For this review, take the finished solid that the model builds, in its own axes (mm). Give positions to 0.01 mm unless a question says otherwise; leave off trailing zeros. Order: outer loops, then holes, each group sorted by start corner. A loop starts at its lowest first (then second) coordinate and runs counter-clockwise, first axis right, second up. Notation, with made-up numbers: (49, 33) - (88, 33) arc R12 ccw to (88, 54) - close; hole circle Ø8 at (63, 44). An arc over 180 degrees is marked (long way). Use a Markdown table: item, result. Add a question column.
1) Clearance check with flat-ended pins moving along their axes: P1, Ø1.5, axis at x = -461, z = 1, coming from the -Y side; P2, Ø0.9, axis at y = 46.5, z = 2, coming from the +X side. State where each tip first meets the part, or that it passes through.
2) Wall thickness on L1, parallel to X at y = -53.5, z = 1.25: over which ranges is the line inside the solid? List them lowest first.
3) We need section A-A on y = 49.5. Write out the cut boundary in (x, z), then the cut area to 3 significant figures.
Autodesk Inventor part; units mm, degrees
ref_plane "YZ Plane" through (0, 0, 0) normal (1, 0, 0) x (0, 1, 0)
ref_plane "XZ Plane" through (0, 0, 0) normal (0, 1, 0) x (-1, 0, 0)
ref_plane "XY Plane" through (0, 0, 0) normal (0, 0, 1) x (1, 0, 0)
sketch "草图1" plane through (0, 0, 0) normal (0, 0, 1) x (1, 0, 0)
  line L0 (477.5, -60) -> (-477.5, -60)
  line L1 (-477.5, -60) -> (-477.5, 60)
  line L2 (-477.5, 60) -> (477.5, 60)
  line L3 (477.5, 60) -> (477.5, -60)
  line L4 (477.5, -60) -> (-477.5, 60) construction
  line L5 (-477.5, -60) -> (477.5, 60) construction
  line L6 (477.5, -40) -> (-477.5, -40)
  line L7 (477.5, 40) -> (-477.5, 40)
  line L8 (-457.5, 40) -> (-457.5, -40)
  line L9 (457.5, 40) -> (457.5, -40)
  line L10 (-455.5, -60) -> (-455.5, 60)
  line L11 (477.5, -39) -> (-477.5, -39)
  line L12 (477.5, 39) -> (-477.5, 39)
  line L13 (-475.5, 59.7487) -> (-475.5, -60)
  line L14 (475.5, 60) -> (475.5, -60)
  line L15 (455.5, 60) -> (455.5, -60)
  point P0 (0, 0)
  point P1 (457.5, -60)
  point P2 (457.5, 60)
  point P3 (-455.5, 40)
  point P4 (-455.5, -40)
  point P5 (457.5, 39)
  point P6 (-457.5, 39)
  point P7 (-457.5, -39)
  point P8 (457.5, -39)
  point P9 (-475.5, 39)
  point P10 (-475.5, -39)
  point P11 (475.5, -39)
  point P12 (475.5, 39)
  point P13 (-455.5, -39)
  point P14 (-455.5, 39)
  point P15 (455.5, -39)
  point P16 (455.5, 39)
  dimension "d0" = 120
  dimension "d1" = 955
  dimension "d4" = 1
  dimension "d5" = 1
  dimension "d6" = 2
  dimension "d7" = 2
  dimension "d8" = 2
  dimension "d9" = 2
extrude "拉伸1" add sketch "草图1" along normal blind 3 contours L0 L10 L6 L15 | L6 L10 L11 L15 | L11 L9 L12 L14 | L15 L12 L9 L11 | L11 L10 L12 L15 | L11 L8 L12 L10 | L12 L10 L7 L15 | L13 L12 L8 L11 | L7 L10 L2 L15
properties part number "内板"
Checked values:
| question | item | result |
|---|---|---|
| 1 | P1 | y = -39 |
| 1 | P2 | x = 455.5 |
| 2 | L1 | -455.5 to 455.5 |
| 3 | outline | (-455.5, 0) - (455.5, 0) - (455.5, 3) - (-455.5, 3) - close |
| 3 | area | 2,730 mm² |
